Read the model definition and answer for the solid it produces. Units are mm, in the model's axes. A direction names the side the tool comes from. Round coordinates to 2 decimals unless told otherwise and drop trailing zeros. Order: outer loops, then holes, each group sorted by start corner. A loop starts at its lowest first (then second) coordinate and runs counter-clockwise, first axis right, second up. Notation, with made-up numbers: (37.5, 17) -> (74.5, 17) arc R20 cw to (74.5, 23) -> close; hole circle Ø3 at (-24.75, 2). An arc over 180 degrees is marked (long way). One line per item, written item: value. Start each with the question number.
1. The mould has two halves that part along X. Classify faces 3 (the face through (-4, -25.4, -8)), 4 (the face through (-2.41, -12.52, 68.19)), 5 (the face through (13.624, -12.522, 3.515)), 6 (the face through (-1.79, -12.52, 43.64)): released by +X, released by -X, zero draft, split by the parting line, or undercut.
2. Section D-D (z = 41) is taken. Give the vertices of the cut face in (x, y), then the cut area to 3 significant figures.
3. Section A-A (x = 0) is taken. Give the vertices of the cut face in (y, z).
4. Section C-C (x = 35.5) is taken. Give the vertices of the cut face in (y, z), then the cut area to 3 significant figures.
5. Section B-B (y = -12.25) is taken. Give the vertices of the cut face in (x, z), then the cut area to 3 significant figures.
6. For faces 1 (the face through (16.247, -12.522, 47.908)), 2 (the face through (-3.081, -12.522, -36.707)), determine the directions among +Z, -Z, +X, -X, +Y, -Y from which every point of the face is accessible in a straight line to the end or side of a thin tool.
7. Consider line 1 (Z direction, x = 41, y = -11.25); line 2 (Z direction, x = 0, y = -21); line 3 (X direction, y = -9.75, z = 53). Determine where each line is inside the solid, lowest interval first.
8. Flat-ended cylindrical pins translate along their axes: pin 1 Ø8 at (x, y) = (9, -17) entering from +Z; pin 2 Ø3 at (x, y) = (18.5, -5) entering from +Z; pin 3 Ø23 at (x, z) = (35.53, -40.59) entering from -Y; pin 4 Ø1 at (x, y) = (-30.5, -2.5) entering from -Z. Find the tip coordinate at first contact, or state that the pin passes through.
from build123d import *

# Parameters (mm, degrees)
F0_R     = 8.24218
F0_R_2   = 7.090267
F0_R_3   = 7.13126
F1_DEPTH = 25.4


with BuildPart() as f1:
    # F0 (on Front) → F1 (new body)
    with BuildSketch(Plane.XZ):
        with BuildLine():
            ThreePointArc((15.015572, 44.421411), (-0.936645, 35.031458), (-15.735387, 46.150886))
            ThreePointArc((-15.735387, 46.150886), (-17.859834, 6.909148), (-47.089189, -19.360076))
            ThreePointArc((-47.089189, -19.360076), (-31.198619, -21.564417), (-23.82385, -35.811597))
            ThreePointArc((-23.82385, -35.811597), (-24.94797, -41.973301), (-28.175494, -47.341107))
            ThreePointArc((-28.175494, -47.341107), (-2.68177, -36.728091), (21.357228, -50.318259))
            ThreePointArc((21.357228, -50.318259), (22.092081, -29.862581), (41.875179, -24.608653))
            ThreePointArc((41.875179, -24.608653), (13.410108, 4.056155), (15.015572, 44.421411))
        make_face()
        with BuildLine():
            ThreePointArc((15.015572, 44.421411), (16.258835, 47.959291), (16.680358, 51.685497))
            ThreePointArc((16.680358, 51.685497), (-2.807352, 68.127915), (-15.735387, 46.150886))
            ThreePointArc((-15.735387, 46.150886), (-0.936645, 35.031458), (15.015572, 44.421411))
        make_face()
        with Locations((0, 51.685497)):
            Circle(F0_R, mode=Mode.SUBTRACT)
        with BuildLine():
            ThreePointArc((-23.82385, -35.811597), (-31.198619, -21.564417), (-47.089189, -19.360076))
            ThreePointArc((-47.089189, -19.360076), (-55.729658, -45.583419), (-28.175494, -47.341107))
            ThreePointArc((-28.175494, -47.341107), (-24.94797, -41.973301), (-23.82385, -35.811597))
        make_face()
        with Locations((-41.273167, -35.811597)):
            Circle(F0_R_2, mode=Mode.SUBTRACT)
        with BuildLine():
            ThreePointArc((52.721042, -40.586339), (49.753447, -30.930781), (41.875179, -24.608653))
            ThreePointArc((41.875179, -24.608653), (22.092081, -29.862581), (21.357228, -50.318259))
            ThreePointArc((21.357228, -50.318259), (40.624096, -57.005833), (52.721042, -40.586339))
        make_face()
        with Locations((35.52927, -40.586339)):
            Circle(F0_R_3, mode=Mode.SUBTRACT)
    extrude(amount=F1_DEPTH)


solid = f1.part
Answer:
1. face 3: zero draft
1. face 4: split by the parting line
1. face 5: released by +X
1. face 6: undercut
2. outline: (-14.22, -25.4) -> (13.51, -25.4) -> (13.51, 0) -> (-14.22, 0) -> close
2. area: 704 mm^2
3. outline: (-25.4, -37.01) -> (0, -37.01) -> (0, 43.44) -> (-25.4, 43.44) -> close; (-25.4, 59.93) -> (0, 59.93) -> (0, 68.37) -> (-25.4, 68.37) -> close
4. outline: (-25.4, -57.78) -> (0, -57.78) -> (0, -47.72) -> (-25.4, -47.72) -> close; (-25.4, -33.46) -> (0, -33.46) -> (0, -21.54) -> (-25.4, -21.54) -> close
4. area: 558 mm^2
5. outline: (-47.09, -19.36) arc R17.45 ccw (long way) to (-28.18, -47.34) arc R31.45 cw to (21.36, -50.32) arc R17.19 ccw (long way) to (41.88, -24.61) arc R50.58 cw to (15.02, 44.42) arc R16.68 ccw to (16.68, 51.69) arc R16.68 ccw (long way) to (-15.74, 46.15) arc R51.4 cw to start; hole circle Ø14.18 at (-41.27, -35.81); hole circle Ø16.48 at (0, 51.69); hole circle Ø14.26 at (35.53, -40.59)
5. area: 5,280 mm^2
6. face 1: +X, +Y, -Y
6. face 2: -Z, +Y, -Y
7. line 1: -56.88 to -45.16, -36.01 to -24.25
7. line 2: -37.01 to 43.44, 59.93 to 68.37
7. line 3: -16.63 to -8.14, 8.14 to 16.63
8. pin 1: z = 67.6
8. pin 2: z = -3.33
8. pin 3: y = -25.4
8. pin 4: z = -49.92
